Input: dimensioned drawing with shaded views. Units: mm. Origin: part minimum x, y, z. A direction names the side the tool comes from. Round coordinates to 2 decimals unless told otherwise and drop trailing zeros. Loops run counter-clockwise (first coordinate to the right, second up) from the corner with the lowest first, then second, coordinate; pieces in that order, holes last. Notation, with made-up numbers: (-1, 38) - (18, 38) arc R23 cw to (18, 59) - close; hole circle Ø10 at (12, 1). An arc over 180 degrees is marked (long way). Answer as a JSON object with one key per item and string values. Group by question number.
Item 1: Reachability of the marked faces 4, 5, 6, 7 and 8 from +Z, -Z, +X, -X, +Y, -Y: full face, straight path, thin tool, end or side. Return the list, or none.
Item 2: Section B-B (y = 27). Count the separate pieces of the cut face and the enclosed holes in it, plus the area to 3 significant figures.
Item 3: First-contact query: pin 1 (5.5 mm diameter, centred on x = 7.62, y = 9.525, fed in from -Z); pin 2 (10 mm diameter, centred on x = 43, y = 8.5, fed in from +Z); pin 3 (8 mm diameter, centred on y = 23.5, z = 31, fed in from +X); pin 4 (1 mm diameter, centred on x = 32, z = 54.5, fed in from -Y). Flat tips, straight axial feed; report the tip coordinate or a pass-through.
Item 4: Section C-C (x = 7.62). Return the cut outline in (y, z).
Item 5: Line query: line 1 (Y direction, x = 43.18, z = 2); line 2 (X direction, y = 24, z = 62); line 3 (Z direction, x = 3, y = 17.5). Output: solid intervals per line, ascending.
Item 6: Draft query along X for the marked faces 1, 2 and 3. Return one class per face: released by +X, released by -X, zero draft, split by the parting line, or undercut.
Item 7: Section A-A (z = 62.23). Return the cut outline in (x, y), plus the area to 3 significant figures.
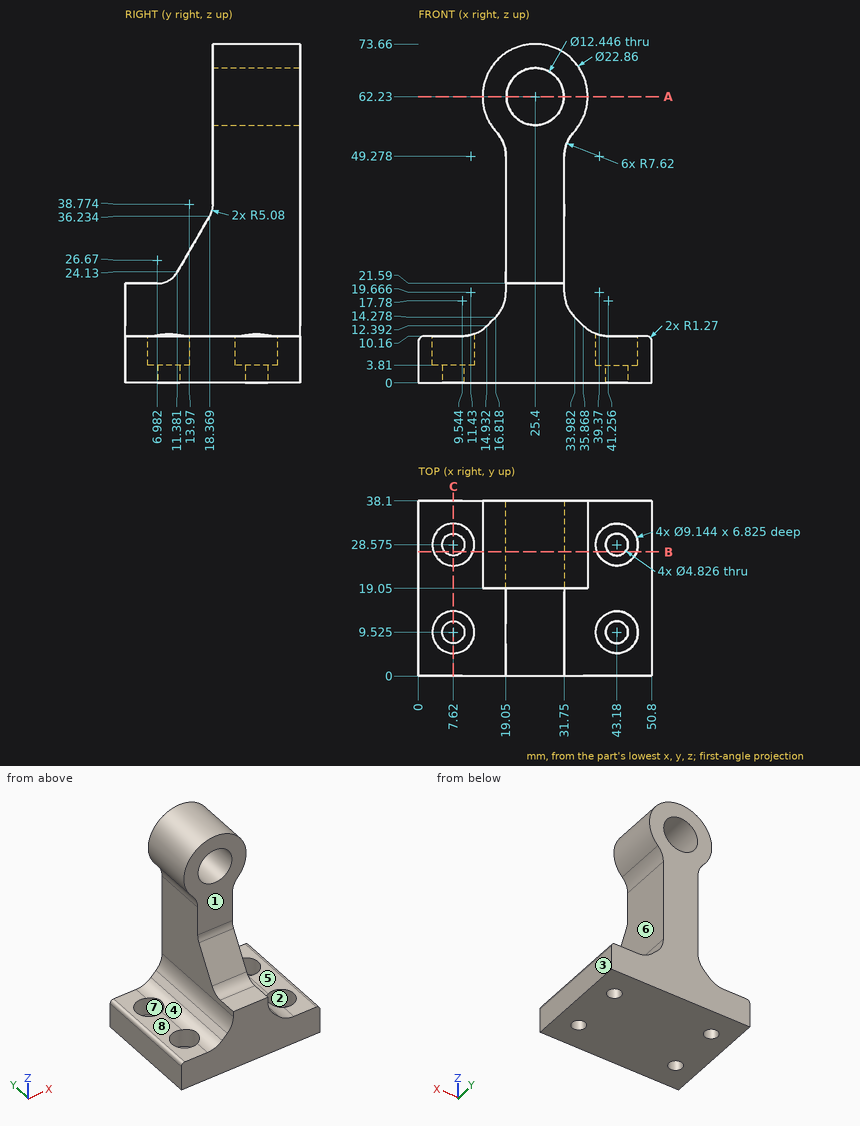
Values:
{
 "1": {"face 4": "-X, +Y, -Y", "face 5": "+Z, +X, +Y, -Y", "face 6": "+X, +Y, -Y", "face 7": "+Z", "face 8": "+Z, -X, +Y, -Y"},
 "2": {"separate pieces": "3", "enclosed holes": "1", "area": "1,240 mm^2"},
 "3": {"pin 1": "stops at z = 0", "pin 2": "stops at z = 10.89", "pin 3": "stops at x = 31.75", "pin 4": "stops at y = 19.05"},
 "4": {"outline": "(0, 0) - (7.11, 0) - (7.11, 3.81) - (4.95, 3.81) - (4.95, 10.16) - (0, 10.16) - close; (11.94, 0) - (26.16, 0) - (26.16, 3.81) - (24, 3.81) - (24, 10.16) - (14.1, 10.16) - (14.1, 3.81) - (11.94, 3.81) - close; (30.99, 0) - (38.1, 0) - (38.1, 10.16) - (33.15, 10.16) - (33.15, 3.81) - (30.99, 3.81) - close"},
 "5": {"line 1": "y = 0 to 7.11, 11.94 to 26.16, 30.99 to 38.1", "line 2": "x = 13.97 to 19.18, 31.62 to 36.83", "line 3": "z = 0 to 10.16"},
 "6": {"face 1": "zero draft", "face 2": "undercut", "face 3": "released by +X"},
 "7": {"outline": "(13.97, 19.05) - (19.18, 19.05) - (19.18, 38.1) - (13.97, 38.1) - close; (31.62, 19.05) - (36.83, 19.05) - (36.83, 38.1) - (31.62, 38.1) - close", "area": "198 mm^2"}
}
